Could you check a few things on this model? Use its own coordinates, in mm. A direction names the side the tool comes from. Round coordinates to 2 decimals unless told otherwise and drop trailing zeros. Loops run counter-clockwise (first coordinate to the right, second up) from the corner with the lowest first, then second, coordinate; pieces in that order, holes last. Notation, with made-up numbers: (23.25, -12) - (80.25, -12) arc R11 ccw to (80.25, 6) - close; hole circle Ø4 at (24.5, 66.25). An arc over 180 degrees is marked (long way). Use one line per item in the form item = value.
```python
from build123d import *

# Parameters (mm, degrees)
F1_R     = 67.5
F1_R_2   = 125
F3_DEPTH = 20
F4_R     = 125
F5_DEPTH = 20


with BuildPart() as f2:
    # F2: sweep along a path in F0
    with BuildLine(Plane.XZ) as f2_path:
        Line((0, 0), (700, 0))
        ThreePointArc((700, 0), (841.421356, -58.578644), (900, -200))
        Line((900, -200), (900, -916))
        ThreePointArc((900, -916), (958.578644, -1057.421356), (1100, -1116))
        Line((1100, -1116), (1600, -1116))
    # F1 (on Right) → F2 (sweep)
    with BuildSketch(Plane.YZ):
        Circle(F1_R)
    sweep(path=f2_path.line)

    # F1 (on Right) → F3 (join)
    with BuildSketch(Plane.YZ):
        Circle(F1_R_2)
        Circle(F1_R, mode=Mode.SUBTRACT)
    extrude(amount=F3_DEPTH)

    # F4 (on face) → F5 (join)
    with BuildSketch(Plane.YZ.offset(1600)):
        with Locations((0, -1116)):
            Circle(F4_R)
    extrude(amount=-F5_DEPTH)


solid = f2.part
```
1. Please list where these lines run through material, in increasing order: line 1 along X through (y, z) = (76.5, -87); line 2 along Z through (x, y) = (513.5, -1); line 3 along Z through (x, y) = (774, 59.5).
Solution:
line_1 = 0 to 20
line_2 = -67.49 to 67.49
line_3 = -49.04 to 19.75
2. For P1, Ø12, axis at y = 44.5, z = -1050.5, coming from the -X side; P2, Ø8, axis at x = 839.5, z = -782.5, coming from the +Y side; P3, Ø8, axis at y = -4.5, z = -252.5, coming from the -X side, each with a flat end and sliding along its axis, tell me the tip position at first contact or that it passes through.
Solution:
P1 = 881.64
P2 = 36.93
P3 = 832.5
3. We'd pull the mould along X, two halves only. Please class faces 4 (the face through (20, 54, -54)), 5 (the face through (1590.14, -124.88, -1110.5)), 6 (the face through (1600, -2, -1114)): +X half, -X half, draft (parallel to the pull), parting line (faces both ways), or undercut.
Solution:
face_4 = undercut
face_5 = draft
face_6 = +X half
4. If we section it at A-A, the plane y = -87: Write out the boundary of the cut face in (x, z).
Solution:
outline = (0, -89.76) - (20, -89.76) - (20, 89.76) - (0, 89.76) - close; (1580, -1205.76) - (1600, -1205.76) - (1600, -1026.24) - (1580, -1026.24) - close
5. On a 3-axis mill with a long thin cutter (end or side, diameter ignored), from which of +Z, -Z, +X, -X, +Y, -Y can I reach the whole of each face in a straight line? I mean faces 1 (the face through (9.86, -124.88, 5.5)), 2 (the face through (364.76, -53.57, -41.07)), 3 (the face through (0, -2, 2)). Say none if no direction works.
Solution:
face_1 = -X
face_2 = none
face_3 = +Z, -Z, -X, +Y, -Y
6. If we section it at B-B, the plane x = 370: Write out the boundary of the cut face in (y, z), plus the area to 3 significant figures.
Solution:
outline = circle Ø135 at (0, 0)
area = 14,300 mm^2
